Input: part model. Units: mm. Frame: model coordinates. A direction names the side the tool comes from. Round coordinates to 2 decimals unless told otherwise and drop trailing zeros. One line per question, with ' | ' between items. Start each with the question number.
from build123d import *

# Parameters (mm, degrees)
F0_W      = 1047.75
F0_H      = 317.5
F1_DEPTH  = 19.05
F2_W      = 19.05
F2_H      = 317.5
F3_DEPTH  = 9.525
F4_W      = 19.05
F4_H      = 317.5
F5_DEPTH  = 9.525
F6_W      = 19.05
F6_H      = 317.5
F7_DEPTH  = 9.525
F8_W      = 19.05
F8_H      = 317.5
F9_DEPTH  = 9.525
F10_W     = 19.05
F10_H     = 317.5
F11_DEPTH = 9.525
F12_W     = 19.05
F12_H     = 317.5
F13_DEPTH = 9.525


with BuildPart() as f1:
    # F0 (on Front) → F1 (new body)
    with BuildSketch(Plane.XZ):
        with Locations((523.875, 158.75)):
            Rectangle(F0_W, F0_H)
    extrude(amount=F1_DEPTH)

    # F2 (on face) → F3 (cut)
    with BuildSketch(Plane.XZ.offset(19.05)):
        with Locations((23.600164, 158.75)):
            Rectangle(F2_W, F2_H)
    extrude(amount=-F3_DEPTH, mode=Mode.SUBTRACT)

    # F4 (on face) → F5 (cut)
    with BuildSketch(Plane.XZ.offset(19.05)):
        with Locations((1023.9375, 158.75)):
            Rectangle(F4_W, F4_H)
    extrude(amount=-F5_DEPTH, mode=Mode.SUBTRACT)

    # F6 (on face) → F7 (cut)
    with BuildSketch(Plane.XZ.offset(19.05)):
        with Locations((823.9125, 158.75)):
            Rectangle(F6_W, F6_H)
    extrude(amount=-F7_DEPTH, mode=Mode.SUBTRACT)

    # F8 (on face) → F9 (cut)
    with BuildSketch(Plane.XZ.offset(19.05)):
        with Locations((220.98, 158.75)):
            Rectangle(F8_W, F8_H)
    extrude(amount=-F9_DEPTH, mode=Mode.SUBTRACT)

    # F10 (on face) → F11 (cut)
    with BuildSketch(Plane.XZ.offset(19.05)):
        with Locations((423.8625, 158.75)):
            Rectangle(F10_W, F10_H)
    extrude(amount=-F11_DEPTH, mode=Mode.SUBTRACT)

    # F12 (on face) → F13 (cut)
    with BuildSketch(Plane.XZ.offset(19.05)):
        with Locations((623.8875, 158.75)):
            Rectangle(F12_W, F12_H)
    extrude(amount=-F13_DEPTH, mode=Mode.SUBTRACT)


solid = f1.part
(1) Pull-direction query (X, two-part tool) for faces 3 (the face through (0, -9, 157)), 4 (the face through (517, -9, 317.5)), 5 (the face through (624, -9.525, 161)); classes: released by +X, released by -X, zero draft, split by the parting line, or undercut.
(2) Line query: line 1 along Y through (x, z) = (820.5, 173.5) (3 decimals). Output: solid intervals per line, ascending. Write a range as from..to.
(3) Pin query (flat end, axial travel): P1, Ø4, axis at x = 222, z = 122.5, coming from the -Y side (3 decimals). Return the tip coordinate at first contact, or that it passes through.
(4) Section A-A, the plane y = -14.5. Give the number of separate pieces and of enclosed holes in the cut face, plus the area to 3 significant figures.
(5) Reachability of faces 1 (the face through (824, -9.525, 161)), 2 (the face through (1047.75, -9, 157)) from +Z, -Z, +X, -X, +Y, -Y: full face, straight path, thin tool, end or side. Return the list, or none.
Derived:
1) face 3: released by -X | face 4: zero draft | face 5: undercut
2) line 1: y = -9.525..0
3) P1: stops at y = -9.525
4) separate pieces: 7 | enclosed holes: 0 | area: 296,000 mm²
5) face 1: +Z, -Z, -Y | face 2: +Z, -Z, +X, +Y, -Y
